Design review of the part shown in the three views and the two pictorial views. Dimensions are in mm from the part's minimum x, y and z. A direction names the side the tool comes from. Coordinates: 2 decimals unless noted, no trailing zeros. Order: outer loops, then holes, each group sorted by start corner. A loop starts at its lowest first (then second) coordinate and runs counter-clockwise, first axis right, second up. Notation, with made-up numbers: (2, 80.5) -> (23, 80.5) arc R28 ccw to (23, 104.5) -> close; hole circle Ø7 at (-25.75, 43.5). An arc over 180 degrees is marked (long way). Answer as a JSON object with one key per item and string values. Group by question number.
1) Machinability: for the marked faces 1 and 2, which of the approach directions +Z, -Z, +X, -X, +Y, -Y give a long, thin tool a straight path to every point of the face, cutting with its end or side? Answer none if there is none.
2) Add section D-D, the plane x = 17. Write out the cut boundary in (y, z) (1 decimal).
3) Add section B-B, the plane z = 0.45. Write out the cut boundary in (x, y) (1 decimal).
4) Add section A-A, the plane x = 30.5. Write out the cut boundary in (y, z) (1 decimal).
5) Wall thickness on L1, parallel to Y at x = 32.5, z = 1.75 (1 decimal); L2, parallel to Y at x = 9, z = 1.95 (1 decimal); L3, parallel to X at y = 9, z = 2.6 (1 decimal): over which ranges is each line inside the solid? List them lowest first.
6) Add section C-C, the plane y = 7. Write out the cut boundary in (x, z).
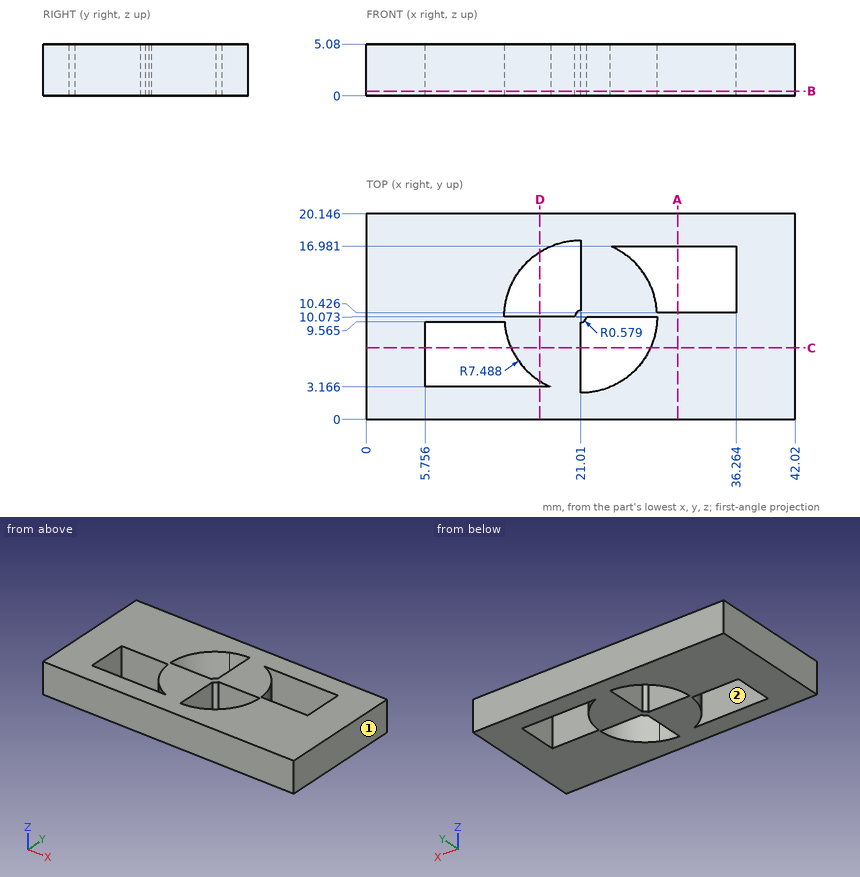
Output values:
{
 "1": {"face 1": "+Z, -Z, +X, +Y, -Y", "face 2": "+Z, -Z"},
 "2": {"outline": "(0, 0) -> (3.2, 0) -> (3.2, 5.1) -> (0, 5.1) -> close; (3.7, 0) -> (10.1, 0) -> (10.1, 5.1) -> (3.7, 5.1) -> close; (16.4, 0) -> (20.1, 0) -> (20.1, 5.1) -> (16.4, 5.1) -> close"},
 "3": {"outline": "(0, 0) -> (42, 0) -> (42, 20.1) -> (0, 20.1) -> close; hole (5.8, 3.2) -> (18.1, 3.2) arc R7.5 cw to (13.5, 9.6) -> (5.8, 9.6) -> close; hole (13.5, 10.1) -> (20.4, 10.1) arc R0.6 cw to (21, 10.7) -> (21, 17.6) arc R7.5 ccw to start; hole (21, 2.6) arc R7.5 ccw to (28.5, 10.1) -> (21.6, 10.1) arc R0.6 cw to (21, 9.5) -> close; hole (23.9, 17) arc R7.5 cw to (28.5, 10.4) -> (36.3, 10.4) -> (36.3, 17) -> close"},
 "4": {"outline": "(0, 0) -> (10.4, 0) -> (10.4, 5.1) -> (0, 5.1) -> close; (17, 0) -> (20.1, 0) -> (20.1, 5.1) -> (17, 5.1) -> close"},
 "5": {"L1": "y = 0 to 10.4, 17 to 20.1", "L2": "y = 0 to 3.2, 9.6 to 20.1", "L3": "x = 0 to 5.8, 13.6 to 21, 28.4 to 42"},
 "6": {"outline": "(0, 0) -> (5.76, 0) -> (5.76, 5.08) -> (0, 5.08) -> close; (14.18, 0) -> (21.01, 0) -> (21.01, 5.08) -> (14.18, 5.08) -> close; (27.84, 0) -> (42.02, 0) -> (42.02, 5.08) -> (27.84, 5.08) -> close"}
}
